Verification items for the finished model (mm, model axes). A direction names the side the tool comes from. Round coordinates to 2 decimals unless told otherwise and drop trailing zeros. Write each loop counter-clockwise with the first axis right and the second up, starting at its lowest first coordinate (ties: lowest second). Pieces come first, ordered by that corner, then holes. Notation, with made-up numbers: M 10,0 L 17,0 A29 ccw 17,35 Z; hole C 57,-36.75 d7. An arc over 180 degrees is marked long. One line per item, written item: value. Start each with the question number.
Item 1: Section check C-C, the plane x = -2.25. Record the cut outline in (y, z).
Item 2: Tool access check on faces 1 (the face through (4.824, -3, 0)), 2 (the face through (0, -3, -2.311)), 3 (the face through (0, 19, 2)), 4 (the face through (-4.824, -3, 0)). Record the directions out of +Z, -Z, +X, -X, +Y, -Y that give a thin tool (end or side, any length) a straight path to the whole face; none if there is none.
Item 3: Section check D-D, the plane y = 13. Record the cut outline in (x, z), then the cut area to 3 significant figures.
Item 4: Gauge pin test, flat ends, axial feed: pin 1 (1 mm diameter, centred on x = 2, y = 13.5, fed in from +Z); pin 2 (1.5 mm diameter, centred on x = 5, z = -1, fed in from +Y); pin 3 (1.8 mm diameter, centred on x = -1.5, y = -3.5, fed in from -Z). Record the tip position at first contact, or that the pin passes through.
Item 5: Thickness scan on probe 1 along Y at (x, z) = (5.25, 2); probe 2 along X at (y, z) = (-3, -0.25); probe 3 along Y at (x, z) = (2, 1.75). Record the ranges inside material, lowest first. Write a range as from..to.
Item 6: Section check A-A, the plane x = 5.5. Record the cut outline in (y, z), then the cut area to 3 significant figures.
Item 7: Section check B-B, the plane y = 26. Record the cut outline in (x, z), then the cut area to 3 significant figures.
from build123d import *

# Parameters (mm, degrees)
SKETCH1_W           = 12.8
SKETCH1_H           = 6.92
BOSS_EXTRUDE1_DEPTH = 10
SKETCH2_R           = 2.88
BOSS_EXTRUDE2_DEPTH = 9
SKETCH3_R           = 1.699009251
BOSS_EXTRUDE3_DEPTH = 10
FILLET1_R           = 1
SKETCH4_W           = 9.648664286
SKETCH4_H           = 4.621814488
BOSS_EXTRUDE4_DEPTH = 6


with BuildPart() as part:
    # Sketch1 → Boss-Extrude1 (new body)
    with BuildSketch(Plane(origin=(0, 0, 0), x_dir=(1, 0, 0), z_dir=(0, 1, 0))):
        Rectangle(SKETCH1_W, SKETCH1_H)
    extrude(amount=BOSS_EXTRUDE1_DEPTH)

    # Sketch2 → Boss-Extrude2 (add)
    with BuildSketch(Plane(origin=(0, 10, 0), x_dir=(1, 0, 0), z_dir=(0, 1, 0))):
        Circle(SKETCH2_R)
    extrude(amount=BOSS_EXTRUDE2_DEPTH)

    # Sketch3 → Boss-Extrude3 (add)
    with BuildSketch(Plane(origin=(0, 19, 0), x_dir=(1, 0, 0), z_dir=(0, 1, 0))):
        Circle(SKETCH3_R)
    extrude(amount=BOSS_EXTRUDE3_DEPTH)

    # Fillet1
    fillet1_edges = [part.edges().sort_by_distance(p)[0] for p in [
        (-1.699009251, 29, 0),
    ]]
    fillet(fillet1_edges, radius=FILLET1_R)

    # Sketch4 → Boss-Extrude4 (add)
    with BuildSketch(Plane.XZ):
        Rectangle(SKETCH4_W, SKETCH4_H)
    extrude(amount=BOSS_EXTRUDE4_DEPTH)


solid = part.part
Response values:
1. outline: M -6,-2.31 L 0,-2.31 L 0,-3.46 L 10,-3.46 L 10,-1.8 L 19,-1.8 L 19,1.8 L 10,1.8 L 10,3.46 L 0,3.46 L 0,2.31 L -6,2.31 Z
2. face 1: +Z, -Z, +X, -Y
2. face 2: -Z, +X, -X, -Y
2. face 3: +Y
2. face 4: +Z, -Z, -X, -Y
3. outline: C 0,0 d5.76
3. area: 26.1 mm2
4. pin 1: stops at z = 2.46
4. pin 2: stops at y = 10
4. pin 3: stops at z = -2.31
5. probe 1: y = 0..10
5. probe 2: x = -4.82..4.82
5. probe 3: y = -6..19
6. outline: M 0,-3.46 L 10,-3.46 L 10,3.46 L 0,3.46 Z
6. area: 69.2 mm2
7. outline: C 0,0 d3.4
7. area: 9.07 mm2
